from build123d import *

# Parameters (mm, degrees)
SKETCH1_W           = 106.68
SKETCH1_H           = 81.28
SKETCH1_R           = 9.8
SKETCH1_R_2         = 9.825
SKETCH1_R_3         = 9.85
SKETCH1_R_4         = 9.875
SKETCH1_R_5         = 9.9
SKETCH1_R_6         = 9.925
SKETCH1_R_7         = 9.95
SKETCH1_R_8         = 9.975
SKETCH1_R_9         = 9.775
SKETCH1_R_10        = 9.75
SKETCH1_R_11        = 9.725
BOSS_EXTRUDE1_DEPTH = 3
BOSS_EXTRUDE2_START = -0.4
SKETCH1_2_W         = 106.68
SKETCH1_2_H         = 81.28
SKETCH1_2_R         = 9.7
SKETCH1_2_R_2       = 9.725
SKETCH1_2_R_3       = 9.75
SKETCH1_2_R_4       = 9.775
SKETCH1_2_R_5       = 9.975
SKETCH1_2_R_6       = 9.95
SKETCH1_2_R_7       = 9.925
SKETCH1_2_R_8       = 9.9
SKETCH1_2_R_9       = 9.875
SKETCH1_2_R_10      = 9.85
SKETCH1_2_R_11      = 9.825
SKETCH1_2_R_12      = 9.8
BOSS_EXTRUDE2_DEPTH = 0.4
FILLET1_R           = 12.7


with BuildPart() as part:
    # Sketch1 → Boss-Extrude1 (new body)
    with BuildSketch(Plane(origin=(0, 0, 0), x_dir=(1, 0, 0), z_dir=(0, 1, 0))):
        with Locations((53.34, 40.64)):
            Rectangle(SKETCH1_W, SKETCH1_H)
        with Locations(Location((15.24, 40.64, 0), (0, 0, 270))):
            Circle(SKETCH1_R, mode=Mode.SUBTRACT)
        with Locations(Location((40.64, 40.64, 0), (0, 0, 270))):
            Circle(SKETCH1_R_2, mode=Mode.SUBTRACT)
        with Locations(Location((66.04, 40.64, 0), (0, 0, 270))):
            Circle(SKETCH1_R_3, mode=Mode.SUBTRACT)
        with Locations(Location((91.44, 40.64, 0), (0, 0, 270))):
            Circle(SKETCH1_R_4, mode=Mode.SUBTRACT)
        with Locations(Location((15.24, 15.24, 0), (0, 0, 270))):
            Circle(SKETCH1_R_5, mode=Mode.SUBTRACT)
        with Locations(Location((40.64, 15.24, 0), (0, 0, 270))):
            Circle(SKETCH1_R_6, mode=Mode.SUBTRACT)
        with Locations(Location((66.04, 15.24, 0), (0, 0, 270))):
            Circle(SKETCH1_R_7, mode=Mode.SUBTRACT)
        with Locations(Location((91.44, 15.24, 0), (0, 0, 270))):
            Circle(SKETCH1_R_8, mode=Mode.SUBTRACT)
        with Locations(Location((91.44, 66.04, 0), (0, 0, 270))):
            Circle(SKETCH1_R_9, mode=Mode.SUBTRACT)
        with Locations(Location((66.04, 66.04, 0), (0, 0, 270))):
            Circle(SKETCH1_R_10, mode=Mode.SUBTRACT)
        with Locations(Location((40.64, 66.04, 0), (0, 0, 270))):
            Circle(SKETCH1_R_11, mode=Mode.SUBTRACT)
    extrude(amount=BOSS_EXTRUDE1_DEPTH)

    # Sketch1_2 → Boss-Extrude2 (add)
    # profile 1 of 13: a face of its own
    with BuildSketch(Plane(origin=(0, 0, 0), x_dir=(1, 0, 0), z_dir=(0, 1, 0)).offset(BOSS_EXTRUDE2_START)):
        with Locations((53.34, 40.64)):
            Rectangle(SKETCH1_2_W, SKETCH1_2_H)
        with Locations((15.24, 66.04)):
            Circle(SKETCH1_2_R, mode=Mode.SUBTRACT)
        with Locations(Location((40.64, 66.04, 0), (0, 0, 270))):
            Circle(SKETCH1_2_R_2, mode=Mode.SUBTRACT)
        with Locations(Location((66.04, 66.04, 0), (0, 0, 270))):
            Circle(SKETCH1_2_R_3, mode=Mode.SUBTRACT)
        with Locations(Location((91.44, 66.04, 0), (0, 0, 270))):
            Circle(SKETCH1_2_R_4, mode=Mode.SUBTRACT)
        with Locations(Location((91.44, 15.24, 0), (0, 0, 270))):
            Circle(SKETCH1_2_R_5, mode=Mode.SUBTRACT)
        with Locations(Location((66.04, 15.24, 0), (0, 0, 270))):
            Circle(SKETCH1_2_R_6, mode=Mode.SUBTRACT)
        with Locations(Location((40.64, 15.24, 0), (0, 0, 270))):
            Circle(SKETCH1_2_R_7, mode=Mode.SUBTRACT)
        with Locations(Location((15.24, 15.24, 0), (0, 0, 270))):
            Circle(SKETCH1_2_R_8, mode=Mode.SUBTRACT)
        with Locations(Location((91.44, 40.64, 0), (0, 0, 270))):
            Circle(SKETCH1_2_R_9, mode=Mode.SUBTRACT)
        with Locations(Location((66.04, 40.64, 0), (0, 0, 270))):
            Circle(SKETCH1_2_R_10, mode=Mode.SUBTRACT)
        with Locations(Location((40.64, 40.64, 0), (0, 0, 270))):
            Circle(SKETCH1_2_R_11, mode=Mode.SUBTRACT)
        with Locations(Location((15.24, 40.64, 0), (0, 0, 270))):
            Circle(SKETCH1_2_R_12, mode=Mode.SUBTRACT)
    # profile 2 of 13: a face of its own
    with BuildSketch(Plane(origin=(0, 0, 0), x_dir=(1, 0, 0), z_dir=(0, 1, 0)).offset(BOSS_EXTRUDE2_START)):
        with Locations(Location((66.04, 40.64, 0), (0, 0, 270))):
            Circle(SKETCH1_2_R_10)
    # profile 3 of 13: a face of its own
    with BuildSketch(Plane(origin=(0, 0, 0), x_dir=(1, 0, 0), z_dir=(0, 1, 0)).offset(BOSS_EXTRUDE2_START)):
        with Locations(Location((66.04, 15.24, 0), (0, 0, 270))):
            Circle(SKETCH1_2_R_6)
    # profile 4 of 13: a face of its own
    with BuildSketch(Plane(origin=(0, 0, 0), x_dir=(1, 0, 0), z_dir=(0, 1, 0)).offset(BOSS_EXTRUDE2_START)):
        with Locations(Location((40.64, 40.64, 0), (0, 0, 270))):
            Circle(SKETCH1_2_R_11)
    # profile 5 of 13: a face of its own
    with BuildSketch(Plane(origin=(0, 0, 0), x_dir=(1, 0, 0), z_dir=(0, 1, 0)).offset(BOSS_EXTRUDE2_START)):
        with Locations(Location((40.64, 15.24, 0), (0, 0, 270))):
            Circle(SKETCH1_2_R_7)
    # profile 6 of 13: a face of its own
    with BuildSketch(Plane(origin=(0, 0, 0), x_dir=(1, 0, 0), z_dir=(0, 1, 0)).offset(BOSS_EXTRUDE2_START)):
        with Locations(Location((15.24, 40.64, 0), (0, 0, 270))):
            Circle(SKETCH1_2_R_12)
    # profile 7 of 13: a face of its own
    with BuildSketch(Plane(origin=(0, 0, 0), x_dir=(1, 0, 0), z_dir=(0, 1, 0)).offset(BOSS_EXTRUDE2_START)):
        with Locations(Location((15.24, 15.24, 0), (0, 0, 270))):
            Circle(SKETCH1_2_R_8)
    # profile 8 of 13: a face of its own
    with BuildSketch(Plane(origin=(0, 0, 0), x_dir=(1, 0, 0), z_dir=(0, 1, 0)).offset(BOSS_EXTRUDE2_START)):
        with Locations(Location((91.44, 15.24, 0), (0, 0, 270))):
            Circle(SKETCH1_2_R_5)
    # profile 9 of 13: a face of its own
    with BuildSketch(Plane(origin=(0, 0, 0), x_dir=(1, 0, 0), z_dir=(0, 1, 0)).offset(BOSS_EXTRUDE2_START)):
        with Locations(Location((91.44, 40.64, 0), (0, 0, 270))):
            Circle(SKETCH1_2_R_9)
    # profile 10 of 13: a face of its own
    with BuildSketch(Plane(origin=(0, 0, 0), x_dir=(1, 0, 0), z_dir=(0, 1, 0)).offset(BOSS_EXTRUDE2_START)):
        with Locations(Location((91.44, 66.04, 0), (0, 0, 270))):
            Circle(SKETCH1_2_R_4)
    # profile 11 of 13: a face of its own
    with BuildSketch(Plane(origin=(0, 0, 0), x_dir=(1, 0, 0), z_dir=(0, 1, 0)).offset(BOSS_EXTRUDE2_START)):
        with Locations(Location((66.04, 66.04, 0), (0, 0, 270))):
            Circle(SKETCH1_2_R_3)
    # profile 12 of 13: a face of its own
    with BuildSketch(Plane(origin=(0, 0, 0), x_dir=(1, 0, 0), z_dir=(0, 1, 0)).offset(BOSS_EXTRUDE2_START)):
        with Locations(Location((40.64, 66.04, 0), (0, 0, 270))):
            Circle(SKETCH1_2_R_2)
    # profile 13 of 13: a face of its own
    with BuildSketch(Plane(origin=(0, 0, 0), x_dir=(1, 0, 0), z_dir=(0, 1, 0)).offset(BOSS_EXTRUDE2_START)):
        with Locations((15.24, 66.04)):
            Circle(SKETCH1_2_R)
    extrude(amount=BOSS_EXTRUDE2_DEPTH)

    # Fillet1
    fillet1_edges = [part.edges().sort_by_distance(p)[0] for p in [
        (0, 1.3, -81.28),
        (106.68, 1.3, -81.28),
        (106.68, 1.3, 0),
        (0, 1.3, 0),
    ]]
    fillet(fillet1_edges, radius=FILLET1_R)


solid = part.part
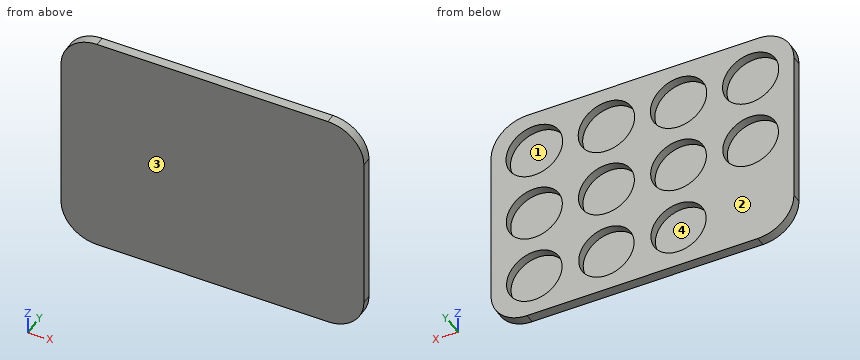
Check sheet for the modelled part. Datum: model origin and axes. Units: mm. Face numbers are marked on the shaded views. A direction names the side the tool comes from. Coordinates: 2 decimals unless noted, no trailing zeros. Write each loop counter-clockwise with the first axis right and the second up, starting at its lowest first coordinate (ties: lowest second). Pieces come first, ordered by that corner, then holes.
Item 1: Cross-section at A-A on y = 1.8. Count the separate pieces of the cut face and the enclosed holes in it, then the cut area to 3 significant figures.
Numbers:
separate pieces: 1
enclosed holes: 11
area: 5,180 mm2
Item 2: Cross-section at C-C on z = -15.24. Record the boundary of the cut face in (x, y) (3 decimals).
Numbers:
outline: (0, -0.4) - (106.68, -0.4) - (106.68, 3) - (101.415, 3) - (101.415, 0) - (81.465, 0) - (81.465, 3) - (75.99, 3) - (75.99, 0) - (56.09, 0) - (56.09, 3) - (50.565, 3) - (50.565, 0) - (30.715, 0) - (30.715, 3) - (25.14, 3) - (25.14, 0) - (5.34, 0) - (5.34, 3) - (0, 3) - close
Item 3: Cross-section at D-D on z = -66.04. Record the boundary of the cut face in (x, y) (3 decimals).
Numbers:
outline: (0, -0.4) - (106.68, -0.4) - (106.68, 3) - (101.215, 3) - (101.215, 0) - (81.665, 0) - (81.665, 3) - (75.79, 3) - (75.79, 0) - (56.29, 0) - (56.29, 3) - (50.365, 3) - (50.365, 0) - (30.915, 0) - (30.915, 3) - (0, 3) - close
Item 4: Depth check by flat-ended pin: pin 1 Ø6 at (x, z) = (91, -16) entering from +Y. Enter the tip coordinate at first touch or a pass-through.
Numbers:
pin 1: stops at y = 0
Item 5: Access from +Z, -Z, +X, -X, +Y, -Y to the whole of each face (thin tool, end or side, straight path). Record for the marked faces 1 and 2.
Numbers:
face 1: +Y
face 2: +Z, -Z, +X, -X, +Y
Item 6: Cross-section at B-B on x = 91.44. Record the boundary of the cut face in (y, z) (3 decimals), then the cut area to 3 significant figures.
Numbers:
outline: (-0.4, -81.28) - (3, -81.28) - (3, -75.815) - (0, -75.815) - (0, -56.265) - (3, -56.265) - (3, -50.515) - (0, -50.515) - (0, -30.765) - (3, -30.765) - (3, -25.215) - (0, -25.215) - (0, -5.265) - (3, -5.265) - (3, 0) - (-0.4, 0) - close
area: 98.6 mm2
Item 7: Mould release check, pull along Z, two halves, no side actions. Record for the marked faces 3 and 4: released by +Z, released by -Z, zero draft, split by the parting line, or undercut.
Numbers:
face 3: zero draft
face 4: undercut
Item 8: Scan lines: probe 1 along X at (y, z) = (1.8, -40.64) (3 decimals); probe 2 along X at (y, z) = (1.4, -15.24) (3 decimals); probe 3 along Z at (x, y) = (47, 2). Record each from-to range of solid material in increasing order.
Numbers:
probe 1: x = 0 to 5.44, 25.04 to 30.815, 50.465 to 56.19, 75.89 to 81.565, 101.315 to 106.68
probe 2: x = 0 to 5.34, 25.14 to 30.715, 50.565 to 56.09, 75.99 to 81.465, 101.415 to 106.68
probe 3: z = -81.28 to -73.4, -58.68 to -48.13, -33.15 to -22.86, -7.62 to 0
